Work out the finished part from the listing and answer in its coordinate system (mm). A direction names the side the tool comes from. Round coordinates to 2 decimals unless told otherwise and drop trailing zeros. Write each loop counter-clockwise with the first axis right and the second up, starting at its lowest first coordinate (ties: lowest second). Pieces come first, ordered by that corner, then holes. Notation, with made-up numbers: (5, 89) - (52, 89) arc R28 ccw to (52, 123) - close; hole circle Ø6 at (82.5, 28). An arc over 180 degrees is marked (long way). Answer as a JSON object with one key per item and string values.
```python
from build123d import *

# Parameters (mm, degrees)
SKETCH1_W           = 35
SKETCH1_H           = 35
BOSS_EXTRUDE1_DEPTH = 20
SKETCH3_R           = 1.5
CUT_EXTRUDE1_DEPTH  = 20
CHAMFER1_SIZE       = 2
SKETCH4_R           = 11.05
BOSS_EXTRUDE2_DEPTH = 2.1
SKETCH5_R           = 7
BOSS_EXTRUDE3_DEPTH = 11.3


with BuildPart() as part:
    # Sketch1 → Boss-Extrude1 (new body)
    with BuildSketch(Plane(origin=(0, 0, 0), x_dir=(1, 0, 0), z_dir=(0, 1, 0))):
        Rectangle(SKETCH1_W, SKETCH1_H)
    extrude(amount=BOSS_EXTRUDE1_DEPTH)

    # Sketch3 → Cut-Extrude1 (cut)
    with BuildSketch(Plane(origin=(0, 20, 0), x_dir=(1, 0, 0), z_dir=(0, 1, 0))):
        with Locations(Location((13, 13, 0), (0, 0, 270))):
            Circle(SKETCH3_R)
        with Locations(Location((13, -13, 0), (0, 0, 270))):
            Circle(SKETCH3_R)
        with Locations(Location((-13, -13, 0), (0, 0, 270))):
            Circle(SKETCH3_R)
        with Locations(Location((-13, 13, 0), (0, 0, 270))):
            Circle(SKETCH3_R)
    extrude(amount=-CUT_EXTRUDE1_DEPTH, mode=Mode.SUBTRACT)

    # Chamfer1
    chamfer1_edges = [part.edges().sort_by_distance(p)[0] for p in [
        (17.5, 10, 17.5),
        (-17.5, 10, 17.5),
        (-17.5, 10, -17.5),
        (17.5, 10, -17.5),
    ]]
    chamfer(chamfer1_edges, length=CHAMFER1_SIZE)

    # Sketch4 → Boss-Extrude2 (add)
    with BuildSketch(Plane(origin=(0, 20, 0), x_dir=(1, 0, 0), z_dir=(0, 1, 0))):
        with Locations(Location((0, 0, 0), (0, 0, 270))):
            Circle(SKETCH4_R)
    extrude(amount=BOSS_EXTRUDE2_DEPTH)

    # Sketch5 → Boss-Extrude3 (add)
    with BuildSketch(Plane(origin=(0, 22.1, 0), x_dir=(1, 0, 0), z_dir=(0, 1, 0))):
        with Locations(Location((0, 0, 0), (0, 0, 270))):
            Circle(SKETCH5_R)
    extrude(amount=BOSS_EXTRUDE3_DEPTH)


solid = part.part
```
Item 1: Consider line 1 along X through (y, z) = (13, -13); line 2 along Y through (x, z) = (-8, 6.5); line 3 along Y through (x, z) = (11, 9). Determine where each line is inside the solid, lowest interval first.
Results found:
{"line 1": "-17.5 to -14.5, -11.5 to 11.5, 14.5 to 17.5", "line 2": "0 to 22.1", "line 3": "0 to 20"}
Item 2: Each of these flat-tipped pins is pushed along its axis until it touches: P1, Ø1.5, axis at x = -12, z = -7, coming from the -Y side; P2, Ø6, axis at x = -12.5, z = 4.5, coming from the +Y side; P3, Ø2.5, axis at x = -13, z = 13, coming from the -Y side; P4, Ø5, axis at x = 13, z = 13, coming from the +Y side. Where does it stop, or does it pass through?
Results found:
{"P1": "y = 0", "P2": "y = 22.1", "P3": "through", "P4": "y = 20"}
Item 3: A cutting plane is placed at C-C (y = 3.5). Write down the section's boundary in (x, z).
Results found:
{"outline": "(-17.5, -15.5) - (-15.5, -17.5) - (15.5, -17.5) - (17.5, -15.5) - (17.5, 15.5) - (15.5, 17.5) - (-15.5, 17.5) - (-17.5, 15.5) - close; hole circle Ø3 at (-13, -13); hole circle Ø3 at (-13, 13); hole circle Ø3 at (13, -13); hole circle Ø3 at (13, 13)"}
Item 4: For faces 4 (the flat face through (0, 10, 17.5)), 5 (the flat face through (-8, 20, -8)), determine the directions among +Z, -Z, +X, -X, +Y, -Y from which every point of the face is accessible in a straight line to the end or side of a thin tool.
Results found:
{"face 4": "+Z, +X, -X, +Y, -Y", "face 5": "+Y"}
Item 5: Determine the mould class of faces 1 (the flat face through (17, 10, 16)), 2 (the cylindrical face through (-6.834, 27.671, -1.517)), 3 (the cylindrical face through (13.07, 10.14, -14.5)) for opening direction X: pulls with the +X half, pulls with the -X half, needs draft (parallel to the pull), parting line crosses it, or undercut.
Results found:
{"face 1": "pulls with the +X half", "face 2": "parting line crosses it", "face 3": "undercut"}
Item 6: A cutting plane is placed at D-D (z = -5). Write down the section's boundary in (x, y).
Results found:
{"outline": "(-17.5, 0) - (17.5, 0) - (17.5, 20) - (9.85, 20) - (9.85, 22.1) - (4.9, 22.1) - (4.9, 33.4) - (-4.9, 33.4) - (-4.9, 22.1) - (-9.85, 22.1) - (-9.85, 20) - (-17.5, 20) - close"}
Item 7: A cutting plane is placed at A-A (z = 13). Write down the section's boundary in (x, y).
Results found:
{"outline": "(-17.5, 0) - (-14.5, 0) - (-14.5, 20) - (-17.5, 20) - close; (-11.5, 0) - (11.5, 0) - (11.5, 20) - (-11.5, 20) - close; (14.5, 0) - (17.5, 0) - (17.5, 20) - (14.5, 20) - close"}
Item 8: A cutting plane is placed at B-B (x = -14). Write down the section's boundary in (y, z).
Results found:
{"outline": "(0, -17.5) - (20, -17.5) - (20, -14.12) - (0, -14.12) - close; (0, -11.88) - (20, -11.88) - (20, 11.88) - (0, 11.88) - close; (0, 14.12) - (20, 14.12) - (20, 17.5) - (0, 17.5) - close"}
